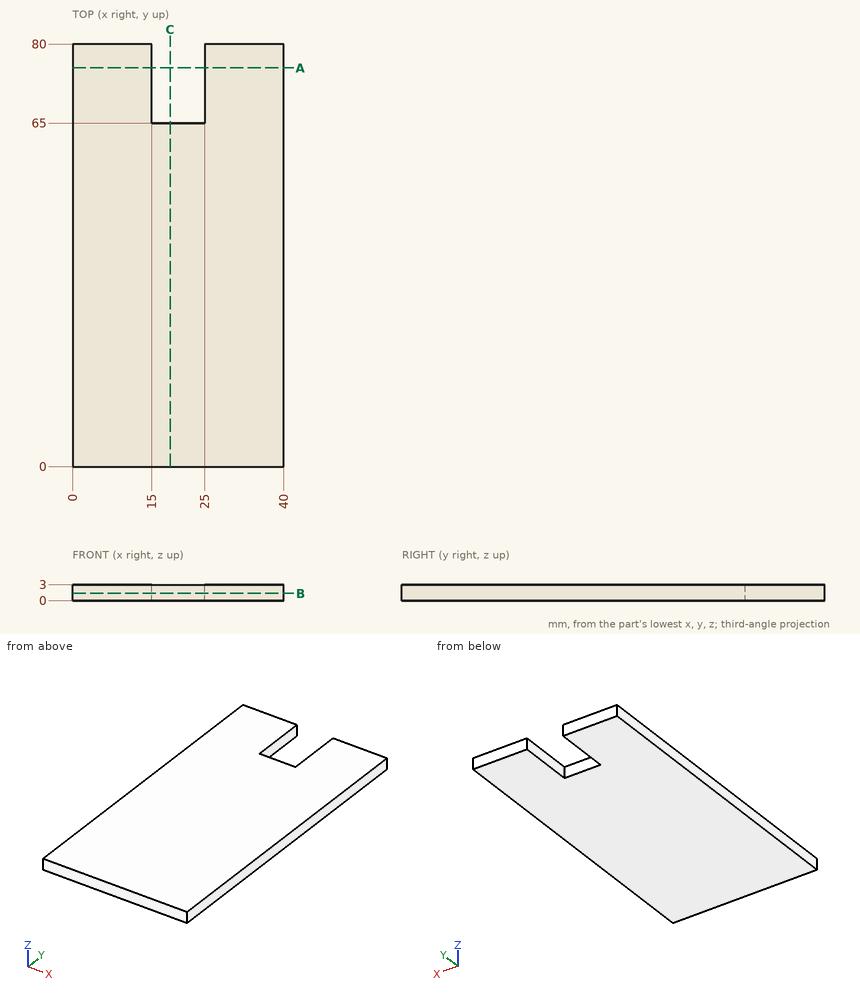
Geometry check sheet. Reference: drawing and pictorial views, mm from the part's lowest x, y, z. Give positions to 0.01 mm unless a question says otherwise; leave off trailing zeros. Write each loop counter-clockwise with the first axis right and the second up, starting at its lowest first coordinate (ties: lowest second). Pieces come first, ordered by that corner, then holes.
Item 1: Scan lines: L1, parallel to X at y = 75.5, z = 1.65; L2, parallel to Y at x = 22.5, z = 0.9. Record each from-to range of solid material in increasing order.
Item 2: Cross-section at A-A (y = 75.5). Enter the section's corners in (x, z), and give its area (3 significant figures).
Item 3: Cross-section at B-B (z = 1.35). Enter the section's corners in (x, y).
Item 4: Gauge pin test, flat end, axial feed: pin 1 (0.9 mm diameter, centred on x = 18.5, z = 2, fed in from +Y). Record the tip position at first contact, or that the pin passes through.
Item 5: Cross-section at C-C (x = 18.5). Enter the section's corners in (y, z).
Report:
1. L1: x = 0 to 15, 25 to 40
1. L2: y = 0 to 65
2. outline: (0, 0) - (15, 0) - (15, 3) - (0, 3) - close; (25, 0) - (40, 0) - (40, 3) - (25, 3) - close
2. area: 90.0 mm2
3. outline: (0, 0) - (40, 0) - (40, 80) - (25, 80) - (25, 65) - (15, 65) - (15, 80) - (0, 80) - close
4. pin 1: stops at y = 65
5. outline: (0, 0) - (65, 0) - (65, 3) - (0, 3) - close
